Work out the finished part from the listing and answer in its coordinate system (mm). Face numbers are marked on the shaded views. A direction names the side the tool comes from. Round coordinates to 2 decimals unless told otherwise and drop trailing zeros. Order: outer loops, then holes, each group sorted by start corner. A loop starts at its lowest first (then second) coordinate and runs counter-clockwise, first axis right, second up.
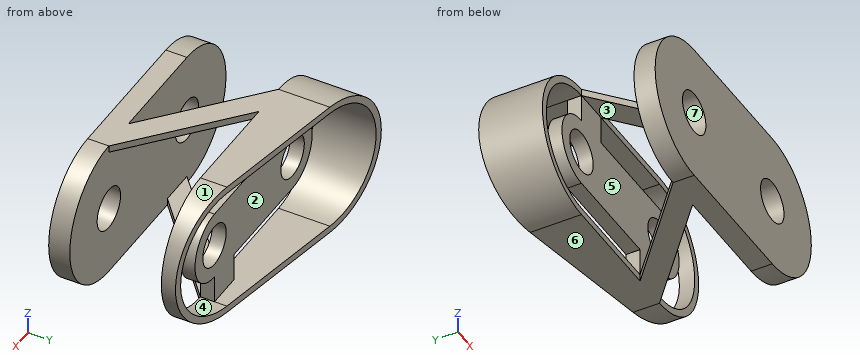
from build123d import *

# Parameters (mm, degrees)
SKETCH1_R               = 15
BOSS_EXTRUDE1_DEPTH     = 15
SKETCH2_R               = 15
SKETCH2_W               = 100
SKETCH2_H               = 5
BOSS_EXTRUDE4_DEPTH     = 10
SKETCH2_7_W             = 100
SKETCH2_7_H             = 5
BOSS_EXTRUDE5_DEPTH     = 40
CUT_EXTRUDE1_DEPTH      = 172.464281995
CUT_EXTRUDE1_DEPTH_BACK = 172.464281995
SKETCH8_OUTSIDE_W       = 253.73
SKETCH8_OUTSIDE_H       = 183.73
LOFT1_START             = 45
LOFT1_DEPTH             = 5
LOFT2_START             = -50
LOFT2_DEPTH             = 5


# Read off the part's stored shape, not the designer's step: Loft1, Loft2
with BuildPart() as part:
    # Sketch1 → Boss-Extrude1 (new body)
    with BuildSketch(Plane(origin=(0, 0, 0), x_dir=(1, 0, 0), z_dir=(0, 1, 0))):
        with BuildLine():
            Line((-50, -50), (50, -50))
            ThreePointArc((50, -50), (100, 0), (50, 50))
            Line((50, 50), (-50, 50))
            ThreePointArc((-50, 50), (-100, 0), (-50, -50))
        make_face()
        with Locations(Location((50, 0, 0), (0, 0, 270))):
            Circle(SKETCH1_R, mode=Mode.SUBTRACT)
        with Locations(Location((-50, 0, 0), (0, 0, 270))):
            Circle(SKETCH1_R, mode=Mode.SUBTRACT)
    extrude(amount=BOSS_EXTRUDE1_DEPTH)



with BuildPart() as body_2:
    # Sketch2 → Boss-Extrude4 (new body)
    # profile 1 of 5: a face of its own
    with BuildSketch(Plane(origin=(0, 90, 0), x_dir=(1, 0, 0), z_dir=(0, 1, 0))):
        with BuildLine():
            Line((50, 45), (25, 45))
            Line((25, 45), (25, 25))
            Line((25, 25), (-50, 25))
            ThreePointArc((-50, 25), (-75, 0), (-50, -25))
            Line((-50, -25), (-50, -43.396517183))
            Line((-50, -43.396517183), (-50, -45))
            Line((-50, -45), (-25, -45))
            Line((-25, -45), (-25, -25))
            Line((-25, -25), (50, -25))
            ThreePointArc((50, -25), (75, 0), (50, 25))
            Line((50, 25), (50, 45))
        make_face()
        with Locations(Location((-50, 0, 0), (0, 0, 270))):
            Circle(SKETCH2_R, mode=Mode.SUBTRACT)
        with Locations(Location((50, 0, 0), (0, 0, 270))):
            Circle(SKETCH2_R, mode=Mode.SUBTRACT)
    # profile 2 of 5: a face of its own
    with BuildSketch(Plane(origin=(0, 90, 0), x_dir=(1, 0, 0), z_dir=(0, 1, 0))):
        with Locations((0, 47.5)):
            Rectangle(SKETCH2_W, SKETCH2_H)
    # profile 3 of 5: a face of its own
    with BuildSketch(Plane(origin=(0, 90, 0), x_dir=(1, 0, 0), z_dir=(0, 1, 0))):
        with BuildLine():
            ThreePointArc((-50, 45), (-95, 0), (-50, -45))
            Line((-50, -45), (-50, -50))
            ThreePointArc((-50, -50), (-100, 0), (-50, 50))
            Line((-50, 50), (-50, 45))
        make_face()
    # profile 4 of 5: a face of its own
    with BuildSketch(Plane(origin=(0, 90, 0), x_dir=(1, 0, 0), z_dir=(0, 1, 0))):
        with BuildLine():
            ThreePointArc((50, -45), (95, 0), (50, 45))
            Line((50, 45), (50, 50))
            ThreePointArc((50, 50), (100, 0), (50, -50))
            Line((50, -50), (50, -45))
        make_face()
    # profile 5 of 5: a face of its own
    with BuildSketch(Plane(origin=(0, 90, 0), x_dir=(1, 0, 0), z_dir=(0, 1, 0))):
        with Locations((0, -47.5)):
            Rectangle(SKETCH2_W, SKETCH2_H)
    extrude(amount=-BOSS_EXTRUDE4_DEPTH)

    # Sketch2<7> → Boss-Extrude5 (add)
    with BuildSketch(Plane(origin=(0, 90, 0), x_dir=(1, 0, 0), z_dir=(0, 1, 0))):
        with Locations((0, 47.5)):
            Rectangle(SKETCH2_7_W, SKETCH2_7_H)
        with BuildLine():
            ThreePointArc((50, -45), (95, 0), (50, 45))
            Line((50, 45), (50, 50))
            ThreePointArc((50, 50), (100, 0), (50, -50))
            Line((50, -50), (50, -45))
        make_face()
        with Locations((0, -47.5)):
            Rectangle(SKETCH2_7_W, SKETCH2_7_H)
        with BuildLine():
            ThreePointArc((-50, 45), (-95, 0), (-50, -45))
            Line((-50, -45), (-50, -50))
            ThreePointArc((-50, -50), (-100, 0), (-50, 50))
            Line((-50, 50), (-50, 45))
        make_face()
    extrude(amount=BOSS_EXTRUDE5_DEPTH)

    # Sketch8 outside → Cut-Extrude1 (cut, two sides: drawn at the far end of the back side and taken through both)
    with BuildSketch(Plane.XY.offset(-CUT_EXTRUDE1_DEPTH_BACK)):
        with Locations((0, 65)):
            Rectangle(SKETCH8_OUTSIDE_W, SKETCH8_OUTSIDE_H)
        Polygon((100, 90), (-100, 125.265396142), (-100, 0), (100, 0), align=None, mode=Mode.SUBTRACT)
    extrude(amount=CUT_EXTRUDE1_DEPTH + CUT_EXTRUDE1_DEPTH_BACK, mode=Mode.SUBTRACT)


with BuildPart() as part_1:
    add(part.part)

    add(body_2.part)  # Loft1 merges body 2
    # Loft1 outline → Loft1 (add)
    with BuildSketch(Plane.XY.offset(LOFT1_START)):
        Polygon((-25, 80), (-50, 80), (25, 15), (50, 15), align=None)
    extrude(amount=LOFT1_DEPTH)

    # Loft2 outline → Loft2 (add)
    with BuildSketch(Plane.XY.offset(LOFT2_START)):
        Polygon((-50, 15), (-25, 15), (50, 80), (25, 80), align=None)
    extrude(amount=LOFT2_DEPTH)


solid = part_1.part
Item 1: Given pin 1 (4 mm diameter, centred on y = 13.5, z = -5, fed in from +X); pin 2 (10 mm diameter, centred on y = 91.5, z = -31.5, fed in from -X); pin 3 (5 mm diameter, centred on y = 94, z = -7.5, fed in from +X); pin 4 (2 mm diameter, centred on x = -56, z = 12.5, fed in from +Y), each flat-ended and moving along its own axis, determine where each tip first touches the part or whether it passes through.
Item 2: Find section B-B (x = -17.5). Write down the section's boundary in (y, z).
Item 3: Find section C-C (y = 39). Write down the section's boundary in (x, z).
Item 4: For a pull along Z with two mould halves and no side action, classify the marked faces 4, 5, 6 and 7 as released by +Z, released by -Z, zero draft, split by the parting line, or undercut.
Item 5: Find section D-D (z = -11). State how many separate pieces and enclosed holes the cut face has, plus the area to 3 significant figures.
Item 6: Find section A-A (z = -42). Write down the section's boundary in (x, y).
Item 7: Find the intervals of material crossed by line 1 along X through (y, z) = (3.25, 0); line 2 along X through (y, z) = (86, 0); line 3 along Y through (x, z) = (-34, 18.5), in increasing order.
Item 8: A tool of negligible diameter and unlimited length cuts with its end or side. For the marked faces 1, 2 and 3, from which of +Z, -Z, +X, -X, +Y, -Y can it reach the whole face along a straight path? Write none if from no direction.
Model answer:
1. pin 1: stops at x = 99.91
1. pin 2: stops at x = -92.4
1. pin 3: stops at x = -93.87
1. pin 4: passes through
2. outline: (0, -50) - (15, -50) - (15, 50) - (0, 50) - close; (21.5, -50) - (43.17, -50) - (43.17, -45) - (21.5, -45) - close; (51.83, 45) - (73.5, 45) - (73.5, 50) - (51.83, 50) - close; (80, -50) - (110.72, -50) - (110.72, -45) - (80, -45) - close; (80, -25) - (90, -25) - (90, 25) - (80, 25) - close; (80, 45) - (110.72, 45) - (110.72, 50) - (80, 50) - close
3. outline: (-22.31, -50) - (2.69, -50) - (2.69, -45) - (-22.31, -45) - close; (-2.69, 45) - (22.31, 45) - (22.31, 50) - (-2.69, 50) - close
4. face 4: undercut
4. face 5: zero draft
4. face 6: released by -Z
4. face 7: undercut
5. separate pieces: 8
5. enclosed holes: 0
5. area: 3,680 mm2
6. outline: (-77.13, 0) - (77.13, 0) - (77.13, 15) - (-77.13, 15) - close; (-77.13, 80) - (-66.16, 80) - (-66.16, 119.3) - (-77.13, 121.23) - close; (25, 80) - (50, 80) - (50, 90) - (25, 90) - close; (66.16, 80) - (77.13, 80) - (77.13, 94.03) - (66.16, 95.97) - close
7. line 1: x = -100 to -65, -35 to 35, 65 to 100
7. line 2: x = -100 to -95, -75 to -65, -35 to 35, 65 to 75, 95 to 100
7. line 3: y = 0 to 15, 80 to 90
8. face 1: +X, +Y, -Y
8. face 2: +Y
8. face 3: +X, -X
